Here's how the part is built. I have some questions about the finished solid (model axes, mm). A direction names the side the tool comes from. Round coordinates to 2 decimals unless told otherwise and drop trailing zeros. Loops run counter-clockwise (first coordinate to the right, second up) from the corner with the lowest first, then second, coordinate; pieces in that order, holes last. Notation, with made-up numbers: M 74.5,31 L 93.5,31 A13 ccw 93.5,37 Z; hole C 12.25,68.25 d2. An arc over 180 degrees is marked long. Use a Markdown table: item, result.
from build123d import *

# Parameters (mm, degrees)
SKETCH1_W           = 80
SKETCH1_H           = 80
BOSS_EXTRUDE1_DEPTH = 5
EXTRUDE_THIN1_DEPTH = 55
FILLET1_R           = 40
SKETCH4_R           = 5
BOSS_EXTRUDE2_DEPTH = 15
SKETCH5_R           = 5
BOSS_EXTRUDE3_DEPTH = 15


with BuildPart() as part:
    # Sketch1 → Boss-Extrude1 (new body)
    with BuildSketch(Plane(origin=(0, 0, 0), x_dir=(1, 0, 0), z_dir=(0, 1, 0))):
        Rectangle(SKETCH1_W, SKETCH1_H)
    extrude(amount=BOSS_EXTRUDE1_DEPTH)

    # Sketch3 → Extrude-Thin1 (add)
    with BuildSketch(Plane(origin=(0, 5, 0), x_dir=(1, 0, 0), z_dir=(0, 1, 0))):
        Polygon((-40, 40), (40, 40), (40, -40), (35, -40), (35, 35), (-40, 35), align=None)
    extrude(amount=EXTRUDE_THIN1_DEPTH)

    # Fillet1
    fillet1_edges = [part.edges().sort_by_distance(p)[0] for p in [
        (37.5, 60, 40),
        (-40, 60, -37.5),
        (-40, 2.5, 40),
    ]]
    fillet(fillet1_edges, radius=FILLET1_R)

    # Sketch4 → Boss-Extrude2 (add)
    with BuildSketch(Plane.ZY.offset(-35)):
        with Locations(Location((20, 40, 0), (0, 0, 180))):
            Circle(SKETCH4_R)
    extrude(amount=BOSS_EXTRUDE2_DEPTH)

    # Sketch5 → Boss-Extrude3 (add)
    with BuildSketch(Plane.XY.offset(-35)):
        with Locations(Location((-20, 40, 0), (0, 0, 180))):
            Circle(SKETCH5_R)
    extrude(amount=BOSS_EXTRUDE3_DEPTH)


solid = part.part
1. Imagine slicing it at C-C, the plane x = 13. Write out the boundary of the cut face in (y, z), then the cut area to 3 significant figures.
Answer sheet:
| item | result |
|---|---|
| outline | M 0,-40 L 60,-40 L 60,-35 L 5,-35 L 5,40 L 0,40 Z |
| area | 675 mm2 |
2. Imagine slicing it at D-D, the plane z = 20. Write out the boundary of the cut face in (x, y).
Answer sheet:
| item | result |
|---|---|
| outline | M -34.64,0 L 40,0 L 40,54.64 L 35,54.64 L 35,45 L 20,45 L 20,35 L 35,35 L 35,5 L -34.64,5 Z |
3. Which directions (+Z, -Z, +X, -X, +Y, -Y) give clear straight access to the entire face, cutting with the end or side of a thin tool? Please do faces 4 (the face through (20, 40, 20)), 5 (the face through (27.605, 35.043, 20.651)), 6 (the face through (36, 60, -29)).
Answer sheet:
| item | result |
|---|---|
| face 4 | +Z, -X, +Y |
| face 5 | -X |
| face 6 | +Z, -Z, +X, -X, +Y |
4. We'd pull the mould along X, two halves only. Please class faces 1 (the face through (-40, 4.8, -22.9)), 2 (the face through (-19.349, 35.043, -27.605)), 3 (the face through (-1, 30, -40)): +X half, -X half, draft (parallel to the pull), parting line (faces both ways), or undercut.
Answer sheet:
| item | result |
|---|---|
| face 1 | -X half |
| face 2 | undercut |
| face 3 | draft |
5. I need wall thicknesses on probe 1 along Y at (x, z) = (-23, 1); probe 2 along X at (y, z) = (9, -2); probe 3 along Z at (x, y) = (-14.5, 54). Which ranges of each line are inside material? Lowest first, please. Write a range as from..to.
Answer sheet:
| item | result |
|---|---|
| probe 1 | 0..5 |
| probe 2 | 35..40 |
| probe 3 | -40..-35 |
6. Imagine slicing it at A-A, the plane z = -28. Write out the boundary of the cut face in (x, y).
Answer sheet:
| item | result |
|---|---|
| outline | M -40,0 L 40,0 L 40,60 L 35,60 L 35,5 L -40,5 Z; C -20,40 d10 |
7. For pin 1 Ø1 at (y, z) = (52, -5.5) entering from -X; pin 2 Ø11 at (x, y) = (-18.5, 39.5) entering from +Z; pin 3 Ø11 at (y, z) = (37.5, 19.5) entering from -X; pin 4 Ø12 at (x, z) = (-18.5, 17) entering from -Y, each with a flat end and sliding along its axis, tell me the tip position at first contact or that it passes through.
Answer sheet:
| item | result |
|---|---|
| pin 1 | x = 35 |
| pin 2 | z = -20 |
| pin 3 | x = 20 |
| pin 4 | y = 0 |
8. Imagine slicing it at B-B, the plane y = 52. Write out the boundary of the cut face in (x, z), then the cut area to 3 significant figures.
Answer sheet:
| item | result |
|---|---|
| outline | M -24,-40 L 40,-40 L 40,24 L 35,24 L 35,-35 L -24,-35 Z |
| area | 615 mm2 |
